CAD build for the part. Positions are in the model's coordinates, mm. Face numbers are marked on the shaded views. A direction names the side the tool comes from. Coordinates: 2 decimals unless noted, no trailing zeros. Loops run counter-clockwise (first coordinate to the right, second up) from the corner with the lowest first, then second, coordinate; pieces in that order, holes last. Notation, with made-up numbers: (62.5, 72.5) -> (87.5, 72.5) arc R20 ccw to (87.5, 80.5) -> close; hole circle Ø7 at (68, 79). An arc over 180 degrees is marked (long way). Write each question's results on one line, items separated by ' | '.
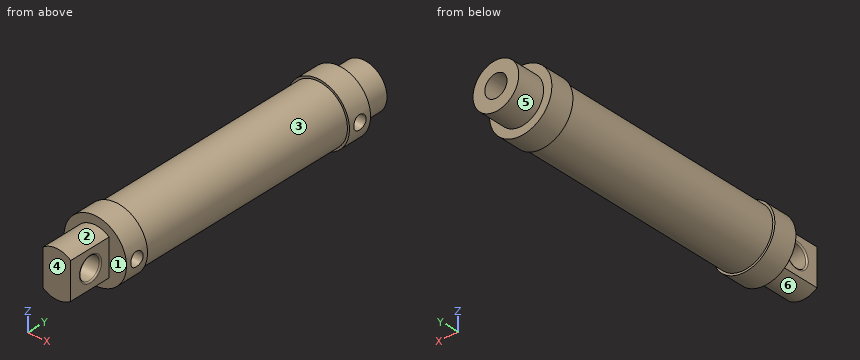
```python
from build123d import *

# Parameters (mm, degrees)
SKETCH_1_R          = 21
SKETCH_1_R_2        = 17.5
EXTRUDE_1_DEPTH     = 163
SKETCH_2_R          = 22.5
EXTRUDE_2_DEPTH     = 17
SKETCH_4_R          = 5
CUT_EXTRUDE_3_DEPTH = 17
EXTRUDE_4_DEPTH     = 31
SKETCH_6_R          = 8
CUT_EXTRUDE_5_DEPTH = 31
FILLET_1_R          = 1
EXTRUDE_START       = 20
SKETCH_7_R          = 16.5
EXTRUDE_6_DEPTH     = 20
CUT_EXTRUDE_9_REACH = 252.033
SKETCH_8_R          = 8


with BuildPart() as part:
    # 草图1 → 拉伸1 (new body)
    with BuildSketch(Plane(origin=(0, 0, 0), x_dir=(1, 0, 0), z_dir=(0, 1, 0))):
        with Locations(Location((0, 0, 0), (0, 0, 270))):
            Circle(SKETCH_1_R)
        with Locations(Location((0, 0, 0), (0, 0, 270))):
            Circle(SKETCH_1_R_2, mode=Mode.SUBTRACT)
    extrude(amount=EXTRUDE_1_DEPTH)

    # 草图2 → 拉伸2 (add)
    with BuildSketch(Plane.XZ):
        with Locations(Location((0, 0, 0), (0, 0, 270))):
            Circle(SKETCH_2_R)
    extrude_2 = extrude(amount=EXTRUDE_2_DEPTH)

    # 草图4 → 拉伸3 (cut)
    with BuildSketch(Plane(origin=(22.5, 0, 0), x_dir=(0, 0, -1), z_dir=(1, 0, 0))):
        with Locations((0, -8.5)):
            Circle(SKETCH_4_R)
    cut_extrude_3 = extrude(amount=-CUT_EXTRUDE_3_DEPTH, mode=Mode.SUBTRACT)

    # 镜向1: 拉伸2, 拉伸3 across plane
    add(extrude_2.mirror(Plane.ZX.offset(81.5)))
    add(cut_extrude_3.mirror(Plane.ZX.offset(81.5)), mode=Mode.SUBTRACT)

    # 草图5 → 拉伸4 (add)
    with BuildSketch(Plane.XZ.offset(17)):
        with BuildLine():
            Line((10, -13.124404748), (10, 13.124404748))
            ThreePointArc((10, 13.124404748), (0, 16.5), (-10, 13.124404748))
            Line((-10, 13.124404748), (-10, -13.124404748))
            ThreePointArc((-10, -13.124404748), (0, -16.5), (10, -13.124404748))
        make_face()
    extrude(amount=EXTRUDE_4_DEPTH)

    # 草图6 → 拉伸5 (cut)
    with BuildSketch(Plane(origin=(10, 0, 0), x_dir=(0, 0, -1), z_dir=(1, 0, 0))):
        with Locations((0, -32)):
            Circle(SKETCH_6_R)
    extrude(amount=-CUT_EXTRUDE_5_DEPTH, mode=Mode.SUBTRACT)

    # 圆角1
    fillet_1_edges = [part.edges().sort_by_distance(p)[0] for p in [
        (-10, -32, 8),
        (10, -32, 8),
    ]]
    fillet(fillet_1_edges, radius=FILLET_1_R)

    # 草图7 → 拉伸6 (add)
    with BuildSketch(Plane(origin=(0, 180, 0), x_dir=(1, 0, 0), z_dir=(0, 1, 0)).offset(EXTRUDE_START)):
        with Locations(Location((0, 0, 0), (0, 0, 270))):
            Circle(SKETCH_7_R)
    extrude(amount=-EXTRUDE_6_DEPTH)

    # 草图8 → 拉伸9 (cut, up to next)
    with BuildSketch(Plane(origin=(0, 200, 0), x_dir=(1, 0, 0), z_dir=(0, 1, 0)), mode=Mode.PRIVATE) as cut_extrude_9_sk1:
        with Locations(Location((0, 0, 0), (0, 0, 270))):
            Circle(SKETCH_8_R)
    cut_extrude_9_tool1 = extrude(cut_extrude_9_sk1.sketch, amount=-CUT_EXTRUDE_9_REACH, mode=Mode.PRIVATE) & part.part
    add(cut_extrude_9_tool1.solids().sort_by_distance((0, 200, 0))[0], mode=Mode.SUBTRACT)


solid = part.part
```
Q1. Which spindle directions (+Z, -Z, +X, -X, +Y, -Y) get a long thin tool onto all of the face, cutting with end or side? Do the marked faces 4, 5 and 6. Say none if no direction does.
Results are:
face 4: +Z, -Z, +X, -X, -Y | face 5: +Y | face 6: -Z, -Y
Q2. Cut at A-A on y = -32. Write the cut outline in (x, z).
Results are:
outline: (-10, -13.12) arc R16.5 ccw to (10, -13.12) -> (10, -9) arc R1 ccw to (9, -8) -> (-9, -8) arc R1 ccw to (-10, -9) -> close; (-10, 9) arc R1 ccw to (-9, 8) -> (9, 8) arc R1 ccw to (10, 9) -> (10, 13.12) arc R16.5 ccw to (-10, 13.12) -> close
Q3. Cut at D-D on y = 78. Write the cut outline in (x, z).
Results are:
outline: circle Ø42 at (0, 0); hole circle Ø35 at (0, 0)
Q4. Wall check: L1, parallel to X at y = 115.5, z = 0; L2, parallel to X at y = 177.5, z = 0; L3, parallel to Y at x = -20, z = -8. Give the ranges that are in metal, low to high. Write a range as from..to.
Results are:
L1: -21..-17.5, 17.5..21 | L2: -22.5..-8, 8..22.5 | L3: -17..0, 163..180
Q5. Drop flat-ended pins along their axis: pin 1 (13 mm diameter, centred on y = -8.5, z = 0, fed in from +X); pin 2 (10 mm diameter, centred on y = -16.5, z = 13.5, fed in from -X); pin 3 (5 mm diameter, centred on x = -0.5, y = 119, fed in from +Z); pin 4 (6 mm diameter, centred on x = -2, z = 0.5, fed in from +Y). Give the stop position or say it passes through.
Results are:
pin 1: x = 22.5 | pin 2: x = -20.83 | pin 3: z = 21 | pin 4: y = 0
Q6. Cut at C-C on z = 0. Give the number of separate pieces and of enclosed holes in the cut face, and give its area (3 significant figures).
Results are:
separate pieces: 3 | enclosed holes: 0 | area: 2,720 mm^2
Q7. Pull direction Y, two halves, no side cores. Call the marked faces 1, 2 and 3: +Y half, -Y half, draft (parallel to the pull), parting line (faces both ways), or undercut.
Results are:
face 1: -Y half | face 2: draft | face 3: undercut
